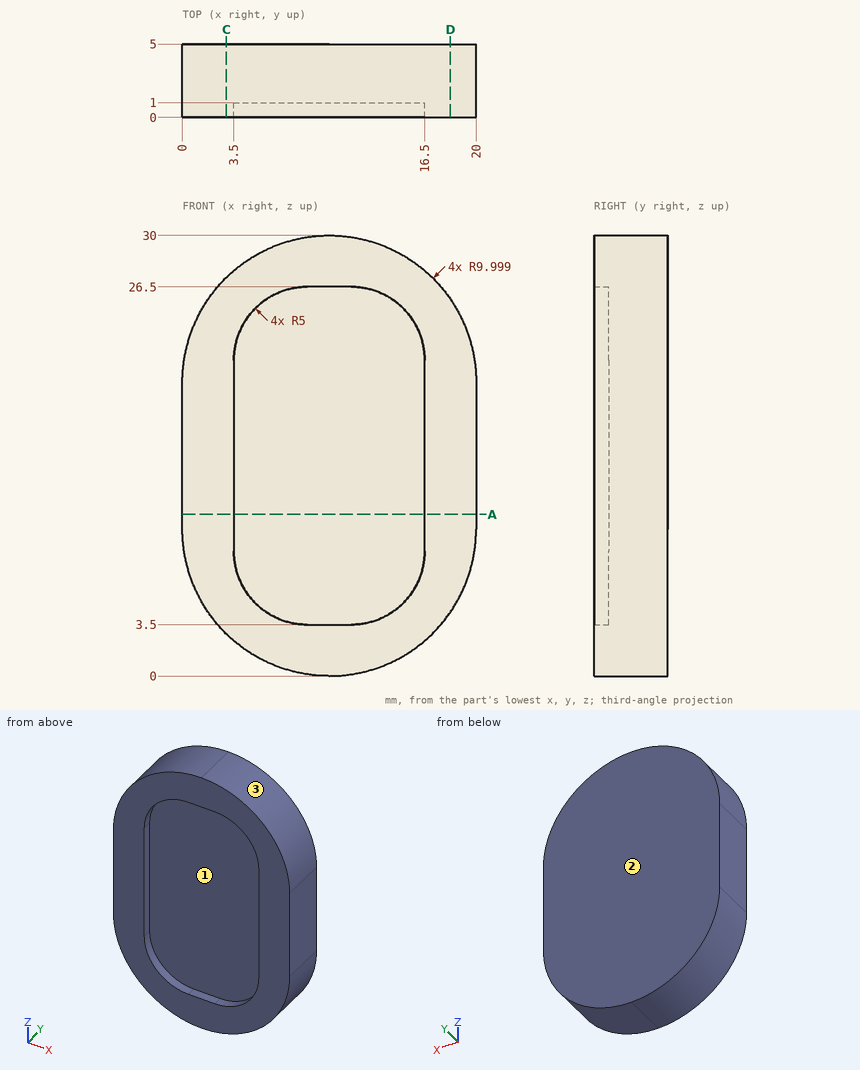
Print and shaded views of the part. All mm, measured from the part's lowest x, y and z. Give positions to 0.01 mm unless a question says otherwise; leave off trailing zeros. Write each loop counter-clockwise with the first axis right and the second up, starting at its lowest first coordinate (ties: lowest second). Pieces come first, ordered by that corner, then holes. Notation, with made-up numbers: (38, -4) - (45, -4) arc R13 ccw to (45, 7) - close; hole circle Ø9 at (37, 3). An arc over 180 degrees is marked (long way). One line per question, with ' | ' between items. Start each with the question number.
(1) Wall check: line 1 along Y through (x, z) = (4.25, 14.75); line 2 along Z through (x, y) = (8.5, 0.75); line 3 along Z through (x, y) = (14.5, 3.1). Give the ranges that are in metal, low to high. Write a range as from..to.
(2) Slice it at C-C on x = 3. Write the cut outline in (y, z).
(3) Slice it at A-A on z = 11. Write the cut outline in (x, y).
(4) Two-plate mould, pull along X, no slides. Class the marked faces 1, 2 and 3: +X half, -X half, draft (parallel to the pull), parting line (faces both ways), or undercut.
(5) Slice it at D-D on x = 18.25. Write the cut outline in (y, z).
(6) Pin check, flat tips, straight feed: P1, Ø1.5, axis at y = 4.5, z = 4, coming from the +X side; P2, Ø1, axis at y = 2.5, z = 4, coming from the +X side; P3, Ø4, axis at x = 12.5, z = 14, coming from the -Y side. Stop position of each tip, or through.
Results below:
1) line 1: 1..5 | line 2: 0.11..3.5, 26.5..29.89 | line 3: 1.07..28.93
2) outline: (0, 2.86) - (5, 2.86) - (5, 27.14) - (0, 27.14) - close
3) outline: (0, 0) - (3.5, 0) - (3.5, 1) - (16.5, 1) - (16.5, 0) - (20, 0) - (20, 5) - (0, 5) - close
4) face 1: undercut | face 2: draft | face 3: +X half
5) outline: (0, 4.35) - (5, 4.35) - (5, 25.65) - (0, 25.65) - close
6) P1: x = 18.51 | P2: x = 18.35 | P3: y = 1
